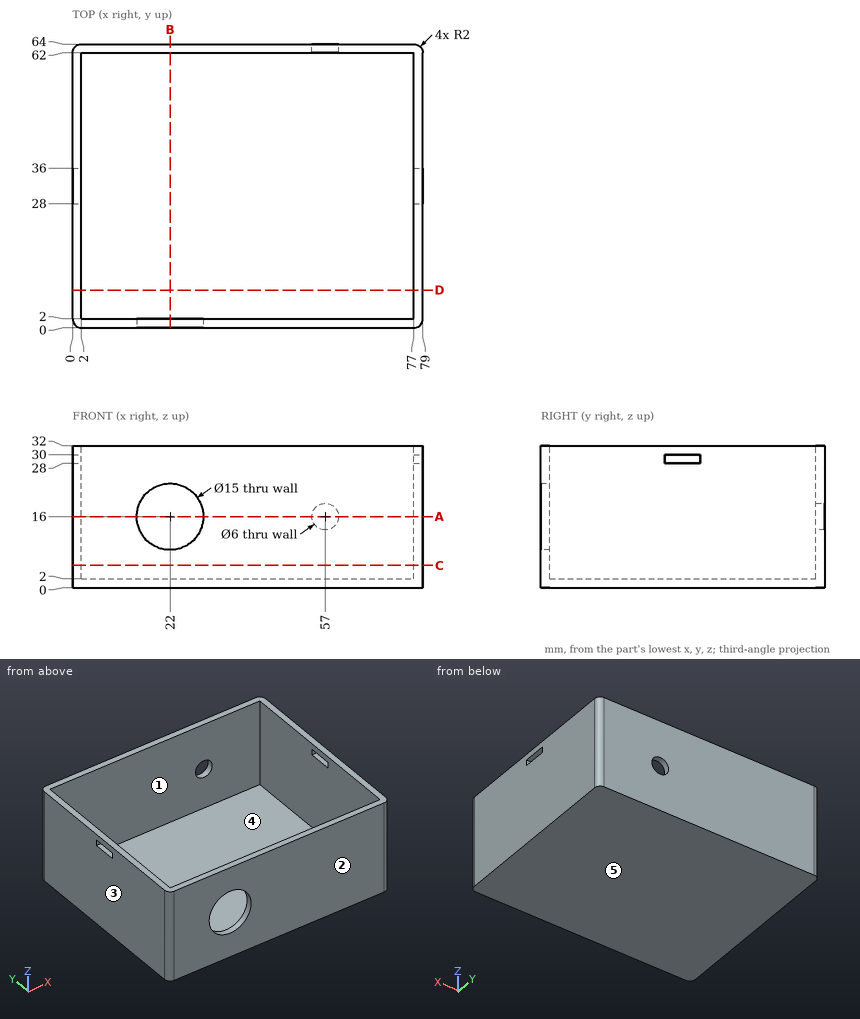
Verification items for this drawing (mm, ordinates from the low corner). A direction names the side the tool comes from. Give positions to 0.01 mm unless a question says otherwise; leave off trailing zeros. Loops run counter-clockwise (first coordinate to the right, second up) from the corner with the lowest first, then second, coordinate; pieces in that order, holes last.
1. Cross-section at A-A on z = 16. Record the cut outline in (x, y), and give its area (3 significant figures).
Derived:
outline: (0, 2) arc R2 ccw to (2, 0) - (14.5, 0) - (14.5, 2) - (2, 2) - (2, 62) - (54, 62) - (54, 64) - (2, 64) arc R2 ccw to (0, 62) - close; (29.5, 0) - (77, 0) arc R2 ccw to (79, 2) - (79, 62) arc R2 ccw to (77, 64) - (60, 64) - (60, 62) - (77, 62) - (77, 2) - (29.5, 2) - close
area: 511 mm2
2. Release check for a two-part mould opening along X. For the marked faces 3, 4 and 5 record: +X half, -X half, draft (parallel to the pull), parting line (faces both ways), or undercut.
Derived:
face 3: -X half
face 4: undercut
face 5: draft
3. Material ranges on probe 1 along Y at (x, z) = (69, 10.5); probe 2 along X at (y, z) = (47.5, 25.5); probe 3 along Z at (x, y) = (57, 62.95), recorded low to high.
Derived:
probe 1: y = 0 to 2, 62 to 64
probe 2: x = 0 to 2, 77 to 79
probe 3: z = 0 to 13, 19 to 32
4. Cross-section at D-D on y = 8.5. Record the cut outline in (x, z).
Derived:
outline: (0, 0) - (79, 0) - (79, 32) - (77, 32) - (77, 2) - (2, 2) - (2, 32) - (0, 32) - close
5. Cross-section at C-C on z = 5. Record the cut outline in (x, y).
Derived:
outline: (0, 2) arc R2 ccw to (2, 0) - (77, 0) arc R2 ccw to (79, 2) - (79, 62) arc R2 ccw to (77, 64) - (2, 64) arc R2 ccw to (0, 62) - close; hole (2, 2) - (77, 2) - (77, 62) - (2, 62) - close
6. Go/stop test with flat-tipped pins: P1, Ø0.6, axis at x = 1, z = 29, coming from the +Y side; P2, Ø0.6, axis at x = 77.5, z = 29, coming from the -Y side; P3, Ø8, axis at x = 42.5, y = 53.5, coming from the +Z side. Record where each tip stops, or that it passes through.
Derived:
P1: stops at y = 63.87
P2: stops at y = 0.01
P3: stops at z = 2
7. Tool access check on the marked faces 1 and 2. Record the directions out of +Z, -Z, +X, -X, +Y, -Y that give a thin tool (end or side, any length) a straight path to the whole face; none if there is none.
Derived:
face 1: +Z
face 2: +Z, -Z, +X, -X, -Y
8. Cross-section at B-B on x = 22. Record the cut outline in (y, z).
Derived:
outline: (0, 0) - (64, 0) - (64, 32) - (62, 32) - (62, 2) - (2, 2) - (2, 8.5) - (0, 8.5) - close; (0, 23.5) - (2, 23.5) - (2, 32) - (0, 32) - close
